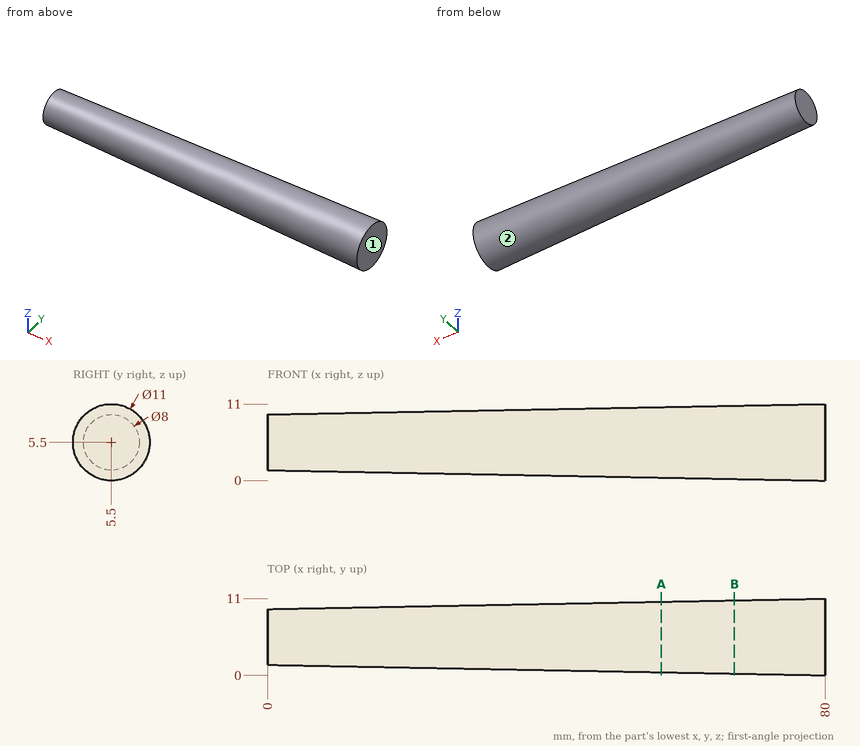
Answer from the drawing. Dimensions are ordinates in mm from the lowest x, y and z of the part. Coordinates: 2 decimals unless noted, no trailing zeros. Loops run counter-clockwise (first coordinate to the right, second up) from the corner with the lowest first, then second, coordinate; pieces in that order, holes last. Notation, with made-up numbers: (-33.75, 72.5) -> (-26.75, 72.5) arc R34 cw to (-26.75, 109.5) -> close; hole circle Ø8 at (25, 81). An arc over 180 degrees is marked (long way). Return JSON: item names as keys, results as strings.
Item 1: Flat-ended cylindrical pins translate along their axes: P1, Ø5, axis at x = 21.5, z = 5.5, coming from the -Y side; P2, Ø5, axis at x = 23.5, y = 8.5, coming from the -Z side; P3, Ø3, axis at x = 36.5, z = 9.5, coming from the -Y side. Find the tip coordinate at first contact, or state that the pin passes through.
Answers:
{"P1": "stops at y = 1.05", "P2": "stops at z = 1.08", "P3": "stops at y = 1.54"}
Item 2: Find section A-A (x = 56.5). Determine the outline of the cut face in (y, z).
Answers:
{"outline": "circle Ø10.12 at (5.5, 5.5)"}
Item 3: Find section B-B (x = 67). Determine the outline of the cut face in (y, z), plus the area to 3 significant figures.
Answers:
{"outline": "circle Ø10.51 at (5.5, 5.5)", "area": "86.8 mm2"}
Item 4: For a pull along X with two mould halves and no side action, classify the marked faces 1 and 2 as +X half, -X half, draft (parallel to the pull), parting line (faces both ways), or undercut.
Answers:
{"face 1": "+X half", "face 2": "-X half"}
Item 5: Find the intervals of material crossed by probe 1 along Y at (x, z) = (53, 3.75); probe 2 along Z at (x, y) = (75.5, 8); probe 3 along Z at (x, y) = (65.5, 9.75), in increasing order.
Answers:
{"probe 1": "y = 0.82 to 10.18", "probe 2": "z = 0.7 to 10.3", "probe 3": "z = 2.46 to 8.54"}
